```python
from build123d import *

# Parameters (mm, degrees)
SKETCH1_R               = 16
BOSS_EXTRUDE1_DEPTH     = 4
SKETCH2_R               = 5
BOSS_EXTRUDE2_DEPTH     = 6
CUT_EXTRUDE1_REACH      = 25.409
SKETCH3_R               = 1.5
SKETCH4_R               = 8
BOSS_EXTRUDE3_DEPTH     = 1
FILLET1_R               = 1
CUT_EXTRUDE2_DEPTH      = 26.159491314
CUT_EXTRUDE2_DEPTH_BACK = 26.159491314
SKETCH5_R               = 2


with BuildPart() as part:
    # Sketch1 → Boss-Extrude1 (new body)
    with BuildSketch(Plane(origin=(0, 0, 0), x_dir=(1, 0, 0), z_dir=(0, 1, 0))):
        with Locations(Location((0, 0, 0), (0, 0, 270))):
            Circle(SKETCH1_R)
    extrude(amount=BOSS_EXTRUDE1_DEPTH)

    # Sketch2 → Boss-Extrude2 (add)
    with BuildSketch(Plane(origin=(0, 4, 0), x_dir=(1, 0, 0), z_dir=(0, 1, 0))):
        with Locations(Location((0, 0, 0), (0, 0, 270))):
            Circle(SKETCH2_R)
    extrude(amount=BOSS_EXTRUDE2_DEPTH)

    # Sketch3 → Cut-Extrude1 (cut, up to next)
    with BuildSketch(Plane(origin=(0, 4, 0), x_dir=(1, 0, 0), z_dir=(0, 1, 0)), mode=Mode.PRIVATE) as cut_extrude1_sk1:
        with Locations(Location((-13, 0, 0), (0, 0, 270))):
            Circle(SKETCH3_R)
    cut_extrude1_tool1 = extrude(cut_extrude1_sk1.sketch, amount=-CUT_EXTRUDE1_REACH, mode=Mode.PRIVATE) & part.part
    # Sketch3 → Cut-Extrude1 (cut, up to next)
    with BuildSketch(Plane(origin=(0, 4, 0), x_dir=(1, 0, 0), z_dir=(0, 1, 0)), mode=Mode.PRIVATE) as cut_extrude1_sk2:
        with Locations(Location((6.5, 11.258330249, 0), (0, 0, 270))):
            Circle(SKETCH3_R)
    cut_extrude1_tool2 = extrude(cut_extrude1_sk2.sketch, amount=-CUT_EXTRUDE1_REACH, mode=Mode.PRIVATE) & part.part
    # Sketch3 → Cut-Extrude1 (cut, up to next)
    with BuildSketch(Plane(origin=(0, 4, 0), x_dir=(1, 0, 0), z_dir=(0, 1, 0)), mode=Mode.PRIVATE) as cut_extrude1_sk3:
        with Locations(Location((6.5, -11.258330249, 0), (0, 0, 270))):
            Circle(SKETCH3_R)
    cut_extrude1_tool3 = extrude(cut_extrude1_sk3.sketch, amount=-CUT_EXTRUDE1_REACH, mode=Mode.PRIVATE) & part.part
    add(cut_extrude1_tool1.solids().sort_by_distance((-13, 4, 0))[0], mode=Mode.SUBTRACT)
    add(cut_extrude1_tool2.solids().sort_by_distance((6.5, 4, -11.25833))[0], mode=Mode.SUBTRACT)
    add(cut_extrude1_tool3.solids().sort_by_distance((6.5, 4, 11.25833))[0], mode=Mode.SUBTRACT)

    # Sketch4 → Boss-Extrude3 (add)
    with BuildSketch(Plane.XZ):
        with Locations(Location((0, 0, 0), (0, 0, 270))):
            Circle(SKETCH4_R)
    extrude(amount=BOSS_EXTRUDE3_DEPTH)

    # Fillet1
    fillet1_edges = [part.edges().sort_by_distance(p)[0] for p in [
        (0, 4, -16),
        (0, 4, -5),
        (0, 10, -5),
    ]]
    fillet(fillet1_edges, radius=FILLET1_R)

    # Sketch5 → Cut-Extrude2 (cut, two sides: drawn at the far end of the back side and taken through both)
    with BuildSketch(Plane(origin=(0, 10, 0), x_dir=(1, 0, 0), z_dir=(0, 1, 0)).offset(-CUT_EXTRUDE2_DEPTH_BACK)):
        with Locations(Location((0, 0, 0), (0, 0, 270))):
            Circle(SKETCH5_R)
    extrude(amount=CUT_EXTRUDE2_DEPTH + CUT_EXTRUDE2_DEPTH_BACK, mode=Mode.SUBTRACT)


solid = part.part
```
Model file for the job. Use its own axes, mm. A direction names the side the tool comes from. Coordinates: 2 decimals unless noted, no trailing zeros. Loops run counter-clockwise (first coordinate to the right, second up) from the corner with the lowest first, then second, coordinate; pieces in that order, holes last. Notation, with made-up numbers: (5.25, 73.5) -> (9.25, 73.5) arc R27 ccw to (9.25, 105.5) -> close; hole circle Ø9 at (46.5, 1.25). An arc over 180 degrees is marked (long way). Answer as a JSON object with one key per item and string values.
Q1. Pull direction X, two halves, no side cores. Call faces 4 (the cylindrical face through (6.57, 2.03, 9.76)), 5 (the flat face through (3.8, 0, -7.3)), 6 (the cylindrical face through (-4.88, 6.97, -1.08)): released by +X, released by -X, zero draft, split by the parting line, or undercut.
Report:
{"face 4": "undercut", "face 5": "zero draft", "face 6": "split by the parting line"}
Q2. Cut at C-C (y = 1). List the corners of the cut face in (x, z).
Report:
{"outline": "circle Ø32 at (0, 0); hole circle Ø3 at (-13, 0); hole circle Ø4 at (0, 0); hole circle Ø3 at (6.5, -11.26); hole circle Ø3 at (6.5, 11.26)"}
Q3. Cut at A-A (z = 0). List the corners of the cut face in (x, y), and give its area (3 significant figures).
Report:
{"outline": "(-16, 0) -> (-14.5, 0) -> (-14.5, 4) -> (-15, 4) arc R1 ccw to (-16, 3) -> close; (-11.5, 0) -> (-8, 0) -> (-8, -1) -> (-2, -1) -> (-2, 10) -> (-4, 10) arc R1 ccw to (-5, 9) -> (-5, 5) arc R1 cw to (-6, 4) -> (-11.5, 4) -> close; (2, -1) -> (8, -1) -> (8, 0) -> (16, 0) -> (16, 3) arc R1 ccw to (15, 4) -> (6, 4) arc R1 cw to (5, 5) -> (5, 9) arc R1 ccw to (4, 10) -> (2, 10) -> close", "area": "148 mm2"}
Q4. Probe probe 1 along X at (y, z) = (6, 0); probe 2 along X at (y, z) = (0.25, 0.5); probe 3 along Y at (x, z) = (-6, 2.5). List the from-to ranges inside material, lowest first.
Report:
{"probe 1": "x = -5 to -2, 2 to 5", "probe 2": "x = -15.99 to -14.41, -11.59 to -1.94, 1.94 to 15.99", "probe 3": "y = -1 to 4"}
Q5. Flat gauge pins, fed straight in: P1, Ø4, axis at y = 3, z = 5.5, coming from the -X side; P2, Ø8, axis at x = -12.5, z = -0.5, coming from the -Y side; P3, Ø2, axis at x = -3, y = 2.5, coming from the +Z side; P4, Ø2.5, axis at x = 6.5, z = 11.26, coming from the +Y side. Where does each tip first touch, or does it go through?
Report:
{"P1": "stops at x = -15.61", "P2": "stops at y = 0", "P3": "stops at z = 15.87", "P4": "passes through"}
Q6. Cut at D-D (x = 6.5). State how many separate pieces and enclosed holes the cut face has, and give its area (3 significant figures).
Report:
{"separate pieces": "3", "enclosed holes": "0", "area": "102 mm2"}
Q7. 3-axis set-ups, long thin cutter, end or side, ignore diameter. For faces 1 (the cylindrical face through (-7.81, -0.49, 1.73)), 2 (the cylindrical face through (5.169, 2.028, -10.566)), 3 (the flat face through (0.2, 4, 6.5)): which of +Z, -Z, +X, -X, +Y, -Y reach the whole face in a straight line?
Report:
{"face 1": "-Y", "face 2": "+Y, -Y", "face 3": "+Y"}
Q8. Cut at B-B (x = 0). List the corners of the cut face in (y, z), and give its area (3 significant figures).
Report:
{"outline": "(-1, -8) -> (0, -8) -> (0, -16) -> (3, -16) arc R1 ccw to (4, -15) -> (4, -6) arc R1 cw to (5, -5) -> (9, -5) arc R1 ccw to (10, -4) -> (10, -2) -> (-1, -2) -> close; (-1, 2) -> (10, 2) -> (10, 4) arc R1 ccw to (9, 5) -> (5, 5) arc R1 cw to (4, 6) -> (4, 15) arc R1 ccw to (3, 16) -> (0, 16) -> (0, 8) -> (-1, 8) -> close", "area": "160 mm2"}
